Work out the finished part from the listing and answer in its coordinate system (mm). A direction names the side the tool comes from. Coordinates: 2 decimals unless noted, no trailing zeros. Loops run counter-clockwise (first coordinate to the right, second up) from the corner with the lowest first, then second, coordinate; pieces in that order, holes last. Notation, with made-up numbers: (38, 27.25) -> (60, 27.25) arc R10 ccw to (60, 35.25) -> close; hole circle Ø6 at (10, 22). An arc over 180 degrees is marked (long way). Answer as CSV lines item,"result".
Autodesk Inventor part; units mm, degrees
ref_plane "YZ Plane" through (0, 0, 0) normal (1, 0, 0) x (0, 1, 0)
ref_plane "XZ Plane" through (0, 0, 0) normal (0, 1, 0) x (-1, 0, 0)
ref_plane "XY Plane" through (0, 0, 0) normal (0, 0, 1) x (1, 0, 0)
sketch "Sketch1" plane through (0, 0, 0) normal (0, 1, 0) x (-1, 0, 0)
  circle A0 centre (0, 0) radius 5.6
  dimension "d0" = 11.2
extrude "Extrusion1" add sketch "Sketch1" along normal blind 12
fillet "Fillet1" radius 2 1 edges at (5.6, 0, 0)
sketch "Sketch2" plane through (0, 12, 0) normal (0, 1, 0) x (1, 0, 0)
  circle A0 centre (0, 0) radius 7
  dimension "d4" = 14
extrude "Extrusion2" add sketch "Sketch2" along normal blind 2
sketch "Sketch3" plane through (0, 0, 0) normal (1, 0, 0) x (0, 1, 0)
  line L0 (14, -7) -> (14, 7)
  line L1 (12, -7) -> (12, 7)
  line L2 (14, 0) -> (35, 0)
  line L3 (35, 0) -> (25.9829, -3.4613)
  line L4 (25.9829, -3.4613) -> (14, -3.4613)
  point P0 (0, 0)
  dimension "d7" = 21
  dimension "d8" = 21
revolve "Revolution1" add sketch "Sketch3" angle 360 about axis through (0, 14, 0) along (0, 1, 0)
fillet "Fillet2" radius 2 3 edges at (5.6, 12, 0) (0, 14, 3.4613) (0, 25.9829, 3.4613)
properties part number "Punta calibración 2_3DPrint"
(1) A cutting plane is placed at A-A, the plane y = 6. Write down the section's boundary in (x, z), and give its area (3 significant figures).
Computed values:
outline,"circle Ø11.2 at (0, 0)"
area,"98.5 mm2"
(2) Flat-ended cylindrical pins translate along their axes: pin 1 Ø3 at (x, y) = (-1, 5) entering from +Z; pin 2 Ø8 at (x, y) = (-5.5, 28.5) entering from -Z; pin 3 Ø2 at (x, z) = (4.5, -2) entering from +Y; pin 4 Ø1.5 at (y, z) = (16.5, 4.5) entering from -X. Find the tip coordinate at first contact, or state that the pin passes through.
Computed values:
pin 1,"z = 5.6"
pin 2,"z = -2.55"
pin 3,"y = 14.72"
pin 4,"through"
(3) Which of the six approach directions +Z, -Z, +X, -X, +Y, -Y give full straight-line access (tool end or side, diameter ignored) to faces 1 (the face through (5.595, 5.989, -0.246)), 2 (the face through (0, 0, 0)), 3 (the face through (4, 14, 4))?
Computed values:
face 1,"-Y"
face 2,"+Z, -Z, +X, -X, -Y"
face 3,"+Y"
(4) Consider line 1 along Z through (x, y) = (4.5, 2); line 2 along Z through (x, y) = (-2.25, 10.5); line 3 along Y through (x, z) = (2.5, 4.5). Determine where each line is inside the solid, lowest interval first.
Computed values:
line 1,"-3.33 to 3.33"
line 2,"-5.17 to 5.17"
line 3,"0.73 to 14.02"
(5) A cutting plane is placed at B-B, the plane y = 30. Write down the section's boundary in (x, z), and give its area (3 significant figures).
Computed values:
outline,"circle Ø3.84 at (0, 0)"
area,"11.6 mm2"
